The listing builds one solid part. Answer for the finished solid, in the listing's coordinates (mm). A direction names the side the tool comes from. Coordinates: 2 decimals unless noted, no trailing zeros. Order: outer loops, then holes, each group sorted by start corner. A loop starts at its lowest first (then second) coordinate and runs counter-clockwise, first axis right, second up. Notation, with made-up numbers: (38, -8.5) -> (83, -8.5) arc R24 cw to (83, 29.5) -> close; hole circle Ø9 at (-31, -26). An arc over 180 degrees is marked (long way). Put each result on its own line as item: value. Start each with the question number.
```python
from build123d import *

# Parameters (mm, degrees)
SKETCH_1_W          = 254.9
SKETCH_1_H          = 133
EXTRUDE_1_DEPTH     = 100
SHELL_1_T           = -5
FILLET_1_R          = 40
FILLET_2_R          = 40
CUT_EXTRUDE_1_DEPTH = 100


with BuildPart() as part:
    # 草图1 → 凸台-拉伸1 (new body)
    with BuildSketch(Plane(origin=(0, 0, 0), x_dir=(1, 0, 0), z_dir=(0, 1, 0))):
        Rectangle(SKETCH_1_W, SKETCH_1_H)
    extrude(amount=EXTRUDE_1_DEPTH)

    # 抽壳1
    shell_1_openings = [part.faces().sort_by_distance(p)[0] for p in [
        (0, 100, 0),
    ]]
    offset(amount=SHELL_1_T, openings=shell_1_openings, kind=Kind.INTERSECTION)

    # 圆角1
    fillet_1_edges = [part.edges().sort_by_distance(p)[0] for p in [
        (122.45, 52.5, 61.5),
        (122.45, 52.5, -61.5),
        (-122.45, 52.5, -61.5),
        (-122.45, 52.5, 61.5),
    ]]
    fillet(fillet_1_edges, radius=FILLET_1_R)

    # 圆角2
    fillet_2_edges = [part.edges().sort_by_distance(p)[0] for p in [
        (127.45, 50, 66.5),
        (-127.45, 50, 66.5),
        (-127.45, 50, -66.5),
        (127.45, 50, -66.5),
    ]]
    fillet(fillet_2_edges, radius=FILLET_2_R)

    # 草图2 → 切除-拉伸1 (cut)
    with BuildSketch(Plane(origin=(0, 5, 0), x_dir=(1, 0, 0), z_dir=(0, 1, 0))):
        with BuildLine():
            Line((-25, 17.5), (25, 17.5))
            ThreePointArc((25, 17.5), (42.5, 0), (25, -17.5))
            Line((25, -17.5), (-25, -17.5))
            ThreePointArc((-25, -17.5), (-42.5, 0), (-25, 17.5))
        make_face()
    extrude(amount=-CUT_EXTRUDE_1_DEPTH, mode=Mode.SUBTRACT)


solid = part.part
```
(1) A tool of negligible diameter and unlimited length cuts with its end or side. For faces 1 (the flat face through (-19, 100, 64)), 2 (the cylindrical face through (-111.044, 51.835, -49.472)), 3 (the cylindrical face through (42.496, 2.535, -0.385)), from which of +Z, -Z, +X, -X, +Y, -Y can it reach the whole face along a straight path? Write none if from no direction.
(2) Find the intervals of material crossed by L1, parallel to Z at x = -80, y = 49.5; L2, parallel to X at y = 61, z = -9; L3, parallel to Z at x = 84.5, y = 85.5, in increasing order.
(3) The part is cut by section A-A on y = 16.5. Determine the outline of the cut face in (x, z), plus the area to 3 significant figures.
(4) The part is cut by section B-B on x = -17. Determine the outline of the cut face in (y, z).
(5) This flat-tipped pin is pushed along its axis until it touches: P1, Ø5, axis at x = 47.5, z = 24, coming from the +Y side. Where does it stop, or does it pass through?
(6) The part is cut by section D-D on x = -68.5. Determine the outline of the cut face in (y, z).
(7) The part is cut by section C-C on z = 0. Determine the outline of the cut face in (x, y).
Worked out:
1. face 1: +Z, -Z, +X, -X, +Y
1. face 2: +Y
1. face 3: +Y, -Y
2. L1: -66.5 to -61.5, 61.5 to 66.5
2. L2: -127.45 to -122.45, 122.45 to 127.45
2. L3: -66.5 to -61.45, 61.45 to 66.5
3. outline: (-127.45, -26.5) arc R40 ccw to (-87.45, -66.5) -> (87.45, -66.5) arc R40 ccw to (127.45, -26.5) -> (127.45, 26.5) arc R40 ccw to (87.45, 66.5) -> (-87.45, 66.5) arc R40 ccw to (-127.45, 26.5) -> close; hole (-122.45, -21.5) arc R40 ccw to (-82.45, -61.5) -> (82.45, -61.5) arc R40 ccw to (122.45, -21.5) -> (122.45, 21.5) arc R40 ccw to (82.45, 61.5) -> (-82.45, 61.5) arc R40 ccw to (-122.45, 21.5) -> close
3. area: 3,780 mm2
4. outline: (0, -66.5) -> (100, -66.5) -> (100, -61.5) -> (5, -61.5) -> (5, -17.5) -> (0, -17.5) -> close; (0, 17.5) -> (5, 17.5) -> (5, 61.5) -> (100, 61.5) -> (100, 66.5) -> (0, 66.5) -> close
5. P1: y = 5
6. outline: (0, -66.5) -> (100, -66.5) -> (100, -61.5) -> (5, -61.5) -> (5, 61.5) -> (100, 61.5) -> (100, 66.5) -> (0, 66.5) -> close
7. outline: (-127.45, 0) -> (-42.5, 0) -> (-42.5, 5) -> (-122.45, 5) -> (-122.45, 100) -> (-127.45, 100) -> close; (42.5, 0) -> (127.45, 0) -> (127.45, 100) -> (122.45, 100) -> (122.45, 5) -> (42.5, 5) -> close
